Part print with two shaded views. Sizes in mm from the minimum x, y, z corner. A direction names the side the tool comes from. Round coordinates to 2 decimals unless told otherwise and drop trailing zeros. Loops run counter-clockwise (first coordinate to the right, second up) from the corner with the lowest first, then second, coordinate; pieces in that order, holes last. Notation, with made-up numbers: M -19,-11 L 16,-11 A10 cw 16,2 Z; hole C -7,82 d1. An arc over 180 degrees is marked long. Use a Markdown table: item, result. Add a question column.
Item 1: Wall check: L1, parallel to Y at x = 33.4, z = 15 (1 decimal); L2, parallel to Y at x = 36.25, z = 15 (3 decimals); L3, parallel to Z at x = 35, y = 30. Give the ranges that are in metal, low to high. Write a range as from..to.
Item 2: Saw through at D-D on z = 2.75. Write the cut outline in (x, y).
Item 3: Saw through at A-A on y = 38.56. Write the cut outline in (x, z).
Item 4: Tool access for the marked faces 4, 5, 6, 7 and 8: list every direction of +Z, -Z, +X, -X, +Y, -Y with a clear straight run to the whole face (end or side of a thin tool).
Item 5: Saw through at B-B on z = 15. Give the number of separate pieces and of enclosed holes in the cut face, then the cut area to 3 significant figures.
Item 6: Two-plate mould, pull along Z, no slides. Class the marked faces 1, 2 and 3: +Z half, -Z half, draft (parallel to the pull), parting line (faces both ways), or undercut.
Item 7: Saw through at C-C on x = 38. Write the cut outline in (y, z) (3 decimals).
Item 8: Pin check, flat tips, straight feed: P1, Ø11, axis at x = 39, y = 6, coming from the -Z side (3 decimals); P2, Ø10, axis at x = 37.5, z = 5, coming from the +Y side; P3, Ø3, axis at y = 21.56, z = 15, coming from the -X side; P4, Ø10, axis at x = 19, z = 13, coming from the -Y side. Stop position of each tip, or through.
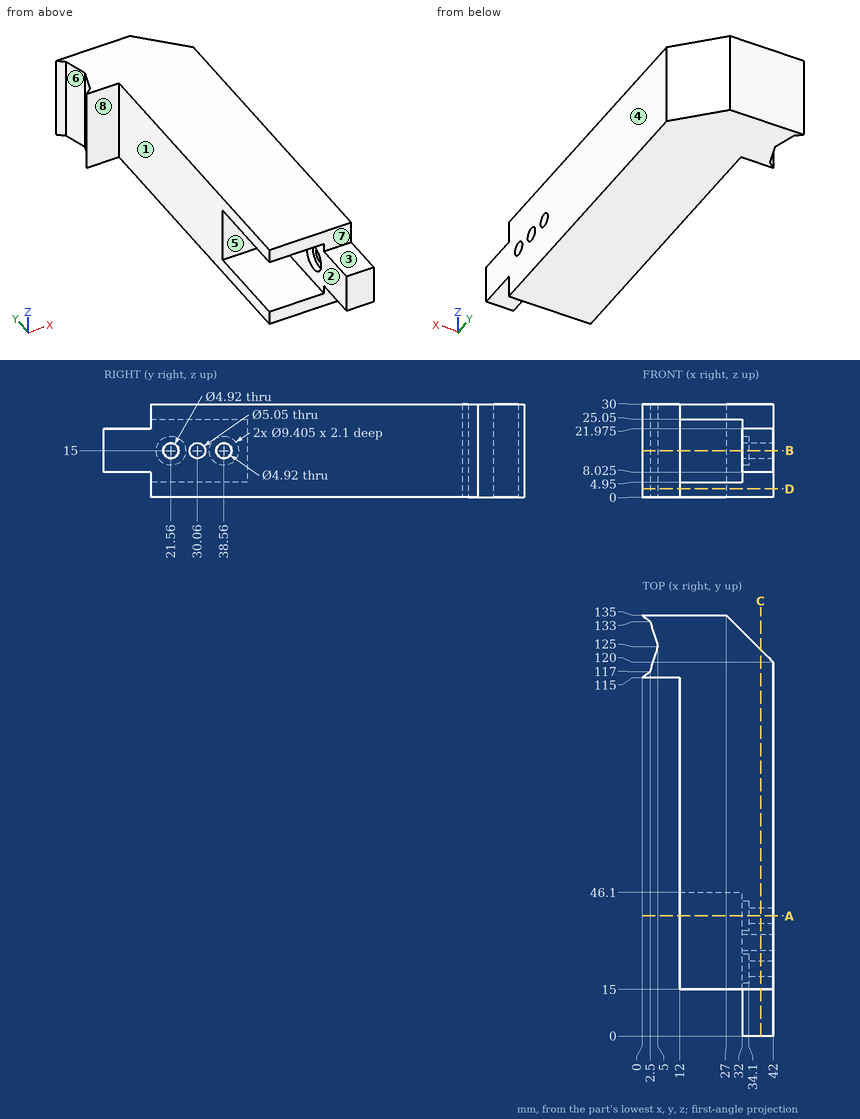
Entries:
| question | item | result |
|---|---|---|
| 1 | L1 | 0..16.9, 26.3..27.5, 32.6..33.9, 43.3..128.6 |
| 1 | L2 | 0..19.1, 24.02..27.535, 32.585..36.1, 41.02..125.75 |
| 1 | L3 | 0..12.48, 17.52..30 |
| 2 | outline | M 0,115 L 12,115 L 12,15 L 42,15 L 42,120 L 27,135 L 0,135 L 2.5,133 L 5,125 L 2.5,117 Z |
| 3 | outline | M 12,0 L 42,0 L 42,12.54 L 34.1,12.54 L 34.1,10.3 L 32,10.3 L 32,4.95 L 12,4.95 Z; M 12,25.05 L 32,25.05 L 32,19.7 L 34.1,19.7 L 34.1,17.46 L 42,17.46 L 42,30 L 12,30 Z |
| 4 | face 4 | +Z, -Z, +X, +Y, -Y |
| 4 | face 5 | -X, -Y |
| 4 | face 6 | +Z, -Z, -X |
| 4 | face 7 | +Z, +X, -X, -Y |
| 4 | face 8 | +Z, -Z, -X, -Y |
| 5 | separate pieces | 4 |
| 5 | enclosed holes | 0 |
| 5 | area | 3,020 mm2 |
| 6 | face 1 | draft |
| 6 | face 2 | undercut |
| 6 | face 3 | +Z half |
| 7 | outline | M 0,8.025 L 15,8.025 L 15,0 L 124,0 L 124,30 L 15,30 L 15,21.975 L 0,21.975 Z; hole C 21.56,15 d4.92; hole C 30.06,15 d5.05; hole C 38.56,15 d4.92 |
| 8 | P1 | z = 8.025 |
| 8 | P2 | y = 129.5 |
| 8 | P3 | through |
| 8 | P4 | y = 46.1 |
